from build123d import *

# Parameters (mm, degrees)
BASPROSKE_W        = 19
BASPROSKE_H        = 17
TOOTHCUT_DEPTH     = 31.643106892
TEETHCUTS_COUNT    = 15
TEETHCUTS_ANGLE    = 336
BORSKE_R           = 0.4
BORE_DEPTH         = 50.0000508
CUT_EXTRUDE1_REACH = 32.615


with BuildPart() as part:
    # BasProSke → Base-Revolve (revolve)
    with BuildSketch(Plane(origin=(0, 0, 0), x_dir=(1, 0, 0), z_dir=(0, 1, 0)), mode=Mode.PRIVATE) as base_revolve_sk:
        with Locations((9.5, 8.5)):
            Rectangle(BASPROSKE_W, BASPROSKE_H)
    revolve(base_revolve_sk.sketch.rotate(Axis((-10, 0, 0), (1, 0, 0)), 180), axis=Axis((-10, 0, 0), (1, 0, 0)))

    # TooCutSke → ToothCut (cut, through all)
    with BuildSketch(Plane(origin=(0, 0, 0), x_dir=(0, 0, -1), z_dir=(1, 0, 0))):
        with BuildLine():
            ThreePointArc((1.050056448, 12.454813626), (0, 12.499), (-1.050056448, 12.454813626))
            ThreePointArc((-1.050056448, 12.454813626), (-1.638118106, 14.809604533), (-3.110934279, 16.73876737))
            ThreePointArc((-3.110934279, 16.73876737), (0, 17.0254), (3.110934279, 16.73876737))
            ThreePointArc((3.110934279, 16.73876737), (1.638118106, 14.809604533), (1.050056448, 12.454813626))
        make_face()
    toothcut = extrude(amount=TOOTHCUT_DEPTH, mode=Mode.SUBTRACT)

    # TeethCuts: ToothCut ×15 about axis
    teethcuts_axis = Axis((-10, 0, 0), (1, 0, 0))
    for i in range(1, TEETHCUTS_COUNT):
        add(toothcut.rotate(teethcuts_axis, i * TEETHCUTS_ANGLE / (TEETHCUTS_COUNT - 1)), mode=Mode.SUBTRACT)

    # BorSke → Bore (cut, symmetric)
    with BuildSketch(Plane(origin=(0, 0, 0), x_dir=(0, 0, -1), z_dir=(1, 0, 0))):
        with Locations(Location((0, 0, 0), (0, 0, 180))):
            Circle(BORSKE_R)
    extrude(amount=BORE_DEPTH, both=True, mode=Mode.SUBTRACT)

    # Sketch1 → Cut-Extrude1 (cut, up to next)
    with BuildSketch(Plane.ZY, mode=Mode.PRIVATE) as cut_extrude1_sk1:
        with BuildLine():
            Line((2.05, -1.907223112), (2.05, 1.907223112))
            ThreePointArc((2.05, 1.907223112), (0, 2.8), (-2.05, 1.907223112))
            Line((-2.05, 1.907223112), (-2.05, -1.907223112))
            ThreePointArc((-2.05, -1.907223112), (0, -2.8), (2.05, -1.907223112))
        make_face()
    cut_extrude1_tool1 = extrude(cut_extrude1_sk1.sketch, amount=-CUT_EXTRUDE1_REACH, mode=Mode.PRIVATE) & part.part
    add(cut_extrude1_tool1.solids().sort_by_distance((0, 0, 0))[0], mode=Mode.SUBTRACT)


solid = part.part
Model file for the job. Use its own axes, mm. A direction names the side the tool comes from. Coordinates: 2 decimals unless noted, no trailing zeros. Loops run counter-clockwise (first coordinate to the right, second up) from the corner with the lowest first, then second, coordinate; pieces in that order, holes last. Notation, with made-up numbers: (-34.75, 5.5) -> (3.25, 5.5) arc R25 ccw to (3.25, 37.5) -> close; hole circle Ø6 at (-29.75, -9.75). An arc over 180 degrees is marked (long way). Use one line per item in the form item = value. Start each with the question number.
(1) Cut at B-B on y = 15.5. Give the cut face in (x, z), and give its area (3 significant figures).
(2) Cut at A-A on z = 0. Give the cut face in (x, y).
(3) Probe probe 1 along Z at (x, y) = (2, -14); probe 2 along Z at (x, y) = (14.75, -5.5); probe 3 along Y at (x, z) = (5.25, -14). List the from-to ranges inside material, lowest first. Write a range as from..to.
(4) Tool access for faces 5 (the cylindrical face through (9.367, 6.147, 13.591)), 6 (the cylindrical face through (9.367, 14.764, 1.617)), 7 (the cylindrical face through (9.367, -3.187, -14.572)), 8 (the cylindrical face through (9.367, -5.987, 13.662)): list every direction of +Z, -Z, +X, -X, +Y, -Y with a clear straight run to the whole face (end or side of a thin tool).
(5) Pull direction Z, two halves, no side cores. Call faces 1 (the cylindrical face through (9.367, -14.844, -1.473)), 2 (the cylindrical face through (9.63, -15.53, 6.92)), 3 (the flat face through (0, 3, 0)), 4 (the cylindrical face through (9.37, -8.84, -12.02)): pulls with the +Z half, pulls with the -Z half, needs draft (parallel to the pull), parting line crosses it, or undercut.
(6) Cut at C-C on z = 14. Give the cut face in (x, y).
(7) Flat gauge pins, fed straight in: pin 1 (8 mm diameter, centred on x = 12.5, y = 9, fed in from +Z); pin 2 (3 mm diameter, centred on x = 15.5, y = -3.5, fed in from +Z); pin 3 (6 mm diameter, centred on x = 13.5, y = -4, fed in from -Z). Where does each tip first touch, or does it go through?
(8) Cut at D-D on y = -14. Give the cut face in (x, z).
Values:
q1.outline = (0, -4.34) -> (19, -4.34) -> (19, -2.03) -> (0, -2.03) -> close; (0, 2.03) -> (19, 2.03) -> (19, 4.34) -> (0, 4.34) -> close
q1.area = 88.0 mm2
q2.outline = (0, -17) -> (19, -17) -> (19, -2.8) -> (0, -2.8) -> close; (0, 2.8) -> (19, 2.8) -> (19, 12.5) -> (0, 12.5) -> close
q3.probe_1 = -7.48..-4.57, -1.62..1.62, 4.57..7.48
q3.probe_2 = -16.09..-11.69, -11.22..11.22, 11.69..16.09
q3.probe_3 = -6..-2.87, -0.16..3.07, 6.58..8.93
q4.face_5 = +Z, +X, -X
q4.face_6 = +X, -X, +Y
q4.face_7 = -Z, +X, -X
q4.face_8 = +X, -X
q5.face_1 = undercut
q5.face_2 = pulls with the +Z half
q5.face_3 = needs draft
q5.face_4 = pulls with the -Z half
q6.outline = (0, -6) -> (19, -6) -> (19, -2.87) -> (0, -2.87) -> close; (0, -0.16) -> (19, -0.16) -> (19, 3.07) -> (0, 3.07) -> close; (0, 6.58) -> (19, 6.58) -> (19, 8.93) -> (0, 8.93) -> close
q7.pin_1 = 14.95
q7.pin_2 = 16.3
q7.pin_3 = -16.3
q8.outline = (0, -7.48) -> (19, -7.48) -> (19, -4.57) -> (0, -4.57) -> close; (0, -1.62) -> (19, -1.62) -> (19, 1.62) -> (0, 1.62) -> close; (0, 4.57) -> (19, 4.57) -> (19, 7.48) -> (0, 7.48) -> close
